from build123d import *

# Parameters (mm, degrees)
F0_R     = 2.1
F1_DEPTH = 500


with BuildPart() as f1:
    # F0 (on Top) → F1 (new body)
    with BuildSketch(Plane.XY):
        with BuildLine():
            Line((10, 4.64), (10, 8.5))
            ThreePointArc((10, 8.5), (9.56066, 9.56066), (8.5, 10))
            Line((8.5, 10), (4.64, 10))
            Line((4.64, 10), (2.84, 8.2))
            Line((2.84, 8.2), (5.49934, 8.2))
            Line((5.49934, 8.2), (5.49934, 6.56))
            Line((5.49934, 6.56), (2.84, 3.90066))
            Line((2.84, 3.90066), (0.25, 3.90066))
            Line((0.25, 3.90066), (0, 3.65066))
            Line((0, 3.65066), (-0.25, 3.90066))
            Line((-0.25, 3.90066), (-2.84, 3.90066))
            Line((-2.84, 3.90066), (-5.49934, 6.56))
            Line((-5.49934, 6.56), (-5.49934, 8.2))
            Line((-5.49934, 8.2), (-2.84, 8.2))
            Line((-2.84, 8.2), (-4.64, 10))
            Line((-4.64, 10), (-8.5, 10))
            ThreePointArc((-8.5, 10), (-9.56066, 9.56066), (-10, 8.5))
            Line((-10, 8.5), (-10, 4.64))
            Line((-10, 4.64), (-8.2, 2.84))
            Line((-8.2, 2.84), (-8.2, 5.49934))
            Line((-8.2, 5.49934), (-6.56, 5.49934))
            Line((-6.56, 5.49934), (-3.90066, 2.84))
            Line((-3.90066, 2.84), (-3.90066, 0.25))
            Line((-3.90066, 0.25), (-3.65066, 0))
            Line((-3.65066, 0), (-3.90066, -0.25))
            Line((-3.90066, -0.25), (-3.90066, -2.84))
            Line((-3.90066, -2.84), (-6.56, -5.49934))
            Line((-6.56, -5.49934), (-8.2, -5.49934))
            Line((-8.2, -5.49934), (-8.2, -2.84))
            Line((-8.2, -2.84), (-10, -4.64))
            Line((-10, -4.64), (-10, -8.5))
            ThreePointArc((-10, -8.5), (-9.56066, -9.56066), (-8.5, -10))
            Line((-8.5, -10), (-4.64, -10))
            Line((-4.64, -10), (-2.84, -8.2))
            Line((-2.84, -8.2), (-5.49934, -8.2))
            Line((-5.49934, -8.2), (-5.49934, -6.56))
            Line((-5.49934, -6.56), (-2.84, -3.90066))
            Line((-2.84, -3.90066), (-0.25, -3.90066))
            Line((-0.25, -3.90066), (0, -3.65066))
            Line((0, -3.65066), (0.25, -3.90066))
            Line((0.25, -3.90066), (2.84, -3.90066))
            Line((2.84, -3.90066), (5.49934, -6.56))
            Line((5.49934, -6.56), (5.49934, -8.2))
            Line((5.49934, -8.2), (2.84, -8.2))
            Line((2.84, -8.2), (4.64, -10))
            Line((4.64, -10), (8.5, -10))
            ThreePointArc((8.5, -10), (9.56066, -9.56066), (10, -8.5))
            Line((10, -8.5), (10, -4.64))
            Line((10, -4.64), (8.2, -2.84))
            Line((8.2, -2.84), (8.2, -5.49934))
            Line((8.2, -5.49934), (6.56, -5.49934))
            Line((6.56, -5.49934), (3.90066, -2.84))
            Line((3.90066, -2.84), (3.90066, -0.25))
            Line((3.90066, -0.25), (3.65066, 0))
            Line((3.65066, 0), (3.90066, 0.25))
            Line((3.90066, 0.25), (3.90066, 2.84))
            Line((3.90066, 2.84), (6.56, 5.49934))
            Line((6.56, 5.49934), (8.2, 5.49934))
            Line((8.2, 5.49934), (8.2, 2.84))
            Line((8.2, 2.84), (10, 4.64))
        make_face()
        Polygon((-6.56934, -7.63), (-6.56934, -8.2), (-8.2, -8.2), (-8.2, -6.56934), (-7.63, -6.56934), align=None, mode=Mode.SUBTRACT)
        Polygon((8.2, -8.2), (6.56934, -8.2), (6.56934, -7.63), (7.63, -6.56934), (8.2, -6.56934), align=None, mode=Mode.SUBTRACT)
        Polygon((-7.63, 6.56934), (-8.2, 6.56934), (-8.2, 8.2), (-6.56934, 8.2), (-6.56934, 7.63), align=None, mode=Mode.SUBTRACT)
        Circle(F0_R, mode=Mode.SUBTRACT)
        Polygon((6.56934, 7.63), (6.56934, 8.2), (8.2, 8.2), (8.2, 6.56934), (7.63, 6.56934), align=None, mode=Mode.SUBTRACT)
    extrude(amount=F1_DEPTH)


solid = f1.part
CAD build for the part. Positions are in the model's coordinates, mm. Coordinates: 2 decimals unless noted, no trailing zeros. Use a Markdown table: item, result. Add a question column.
Item 1: Band-saw the part on A-A, the plane z = 48.5. Give the number of separate pieces and of enclosed holes in the cut face, and give its area (3 significant figures).
Item 2: Flat gauge pins, fed straight in: pin 1 (12 mm diameter, centred on y = 2.5, z = 357, fed in from +X); pin 2 (2 mm diameter, centred on x = 1.5, z = 134.5, fed in from -Y); pin 3 (3 mm diameter, centred on y = 2, z = 311.5, fed in from +X); pin 4 (3 mm diameter, centred on y = -2, z = 131.5, fed in from -X). Where does each tip first touch, or does it go through?
Item 3: Drill centre lines: L1, parallel to Y at x = 8, z = 283; L2, parallel to Y at x = 0, z = 209.5; L3, parallel to X at y = -7.25, z = 130. Where is each one in solid material? Low to high. Write a range as from..to.
Numbers:
| question | item | result |
|---|---|---|
| 1 | separate pieces | 1 |
| 1 | enclosed holes | 5 |
| 1 | area | 161 mm2 |
| 2 | pin 1 | x = 10 |
| 2 | pin 2 | y = -3.9 |
| 2 | pin 3 | x = 8.86 |
| 2 | pin 4 | x = -8.86 |
| 3 | L1 | -10..-8.2, -6.57..-5.5, 5.5..6.57, 8.2..10 |
| 3 | L2 | -3.65..-2.1, 2.1..3.65 |
| 3 | L3 | -10..-8.2, -6.95..-5.5, 5.5..6.95, 8.2..10 |
